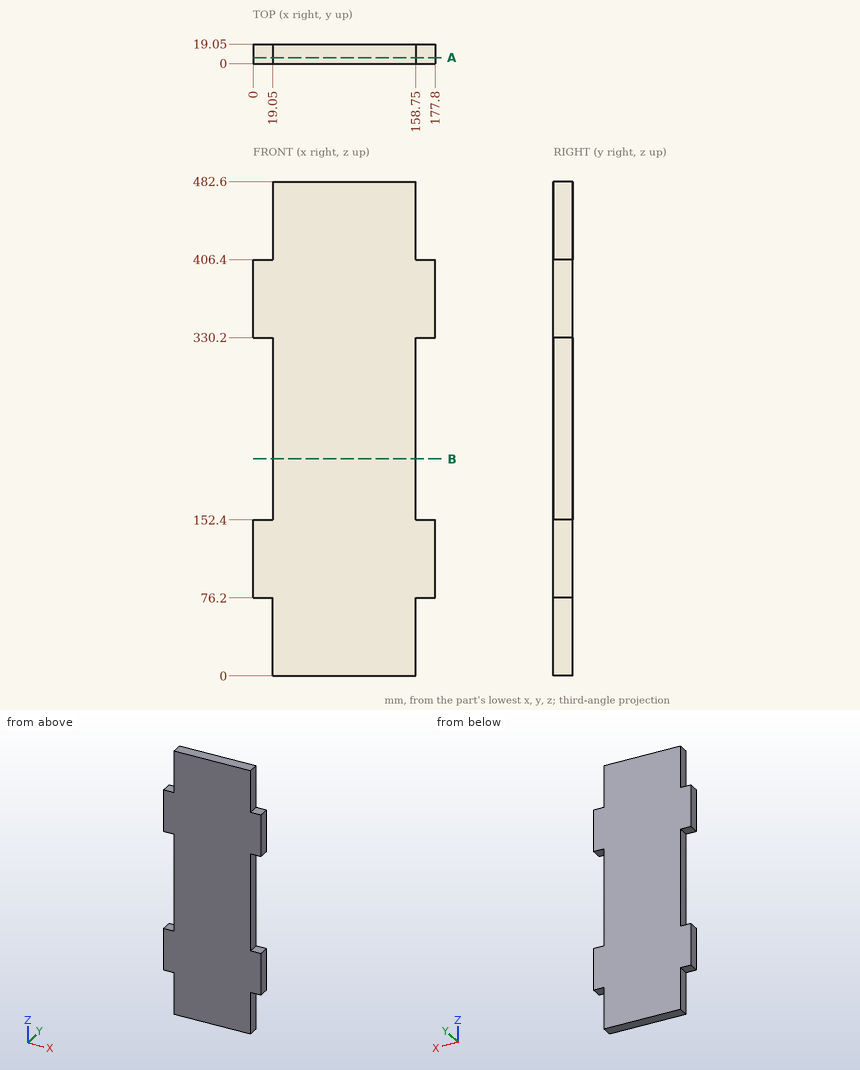
Geometry: see drawing. Coordinates: mm, zero at the bounding-box minimum. Coordinates: 2 decimals unless noted, no trailing zeros. Order: outer loops, then holes, each group sorted by start corner. A loop starts at its lowest first (then second) coordinate and runs counter-clockwise, first axis right, second up. Notation, with made-up numbers: (77, 15) -> (131, 15) arc R16 ccw to (131, 29) -> close; hole circle Ø9 at (-6, -9). An arc over 180 degrees is marked (long way). Write each question's results on one line, items separated by ' | '. Start each with the question number.
1) Cut plane B-B, the plane z = 212. Output: boundary loops of the cut face in (x, y).
2) First-contact query: pin 1 (5.5 mm diameter, centred on y = 8.5, z = 40.5, fed in from -X); pin 2 (5.5 mm diameter, centred on x = 166, y = 8, fed in from +Z); pin 3 (5.5 mm diameter, centred on y = 7.5, z = 463, fed in from +X). Flat tips, straight axial feed; report the tip coordinate or a pass-through.
3) Cut plane A-A, the plane y = 5.75. Output: boundary loops of the cut face in (x, z), and give its area (3 significant figures).
4) Material intervals for line 1 along X through (y, z) = (10.5, 199.5), sorted ascending.
Checks:
1) outline: (19.05, 0) -> (158.75, 0) -> (158.75, 19.05) -> (19.05, 19.05) -> close
2) pin 1: x = 19.05 | pin 2: z = 406.4 | pin 3: x = 158.75
3) outline: (0, 76.2) -> (19.05, 76.2) -> (19.05, 0) -> (158.75, 0) -> (158.75, 76.2) -> (177.8, 76.2) -> (177.8, 152.4) -> (158.75, 152.4) -> (158.75, 330.2) -> (177.8, 330.2) -> (177.8, 406.4) -> (158.75, 406.4) -> (158.75, 482.6) -> (19.05, 482.6) -> (19.05, 406.4) -> (0, 406.4) -> (0, 330.2) -> (19.05, 330.2) -> (19.05, 152.4) -> (0, 152.4) -> close | area: 73,200 mm^2
4) line 1: 19.05 to 158.75
